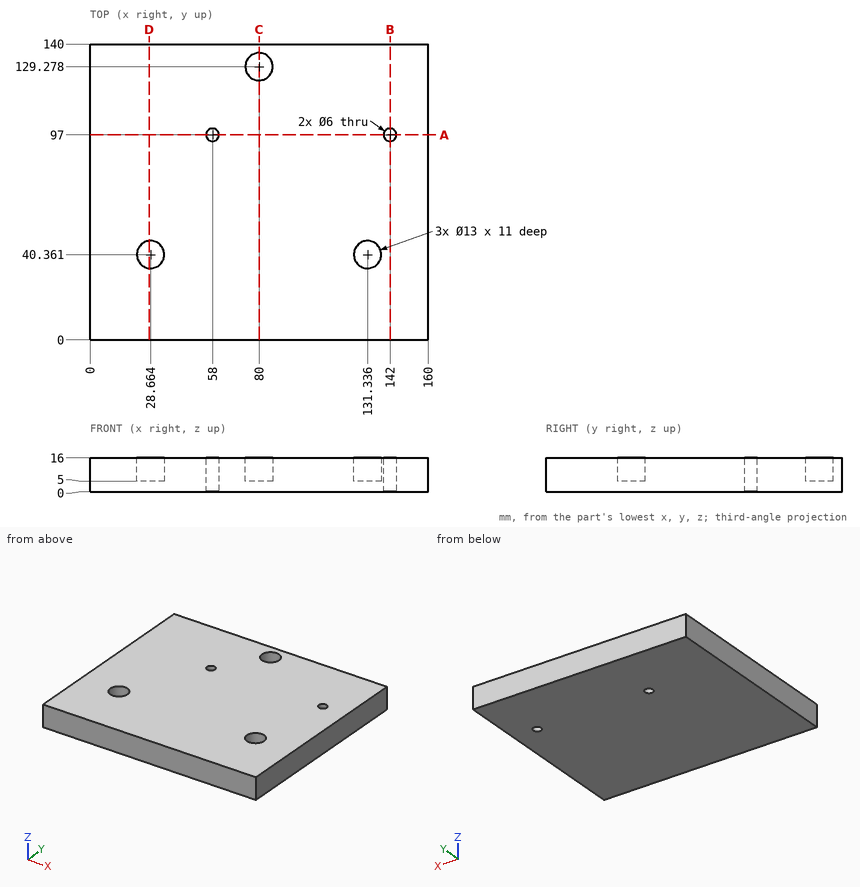
The figure shows three views and two pictorial views of one solid part (mm, origin at its lowest corner). Answer the questions. Give positions to 0.01 mm unless a question says otherwise; leave off trailing zeros. Loops run counter-clockwise (first coordinate to the right, second up) from the corner with the lowest first, then second, coordinate; pieces in that order, holes last. Notation, with made-up numbers: (-0.5, 10) - (18.5, 10) arc R32 cw to (18.5, 38) - close; hole circle Ø2 at (-28, 28). An arc over 180 degrees is marked (long way). Use one line per item in the form item = value.
1. Find the intervals of material crossed by line 1 along X through (y, z) = (97, 8.5); line 2 along X through (y, z) = (41, 7.25) (1 decimal); line 3 along Y through (x, z) = (58, 7.75), in increasing order. Write a range as [from, to].
Calculated:
line_1 = [0, 55], [61, 139], [145, 160]
line_2 = [0, 22.2], [35.1, 124.9], [137.8, 160]
line_3 = [0, 94], [100, 140]
2. Section B-B on x = 142 is taken. Give the vertices of the cut face in (y, z).
Calculated:
outline = (0, 0) - (94, 0) - (94, 16) - (0, 16) - close; (100, 0) - (140, 0) - (140, 16) - (100, 16) - close
3. Section C-C on x = 80 is taken. Give the vertices of the cut face in (y, z).
Calculated:
outline = (0, 0) - (140, 0) - (140, 16) - (135.78, 16) - (135.78, 5) - (122.78, 5) - (122.78, 16) - (0, 16) - close
4. Section A-A on y = 97 is taken. Give the vertices of the cut face in (x, z), then the cut area to 3 significant figures.
Calculated:
outline = (0, 0) - (55, 0) - (55, 16) - (0, 16) - close; (61, 0) - (139, 0) - (139, 16) - (61, 16) - close; (145, 0) - (160, 0) - (160, 16) - (145, 16) - close
area = 2,370 mm^2
5. Given pin 1 Ø10.5 at (x, y) = (26, 43) entering from +Z; pin 2 Ø10.5 at (x, y) = (28.66, 40.36) entering from +Z; pin 3 Ø3.5 at (x, y) = (142, 97) entering from +Z, each flat-ended and moving along its own axis, determine where each tip first touches the part or whether it passes through.
Calculated:
pin_1 = 16
pin_2 = 5
pin_3 = through
6. Section D-D on x = 28 is taken. Give the vertices of the cut face in (y, z) (1 decimal), then the cut area to 3 significant figures.
Calculated:
outline = (0, 0) - (140, 0) - (140, 16) - (46.8, 16) - (46.8, 5) - (33.9, 5) - (33.9, 16) - (0, 16) - close
area = 2,100 mm^2
